Input: dimensioned drawing with shaded views. Units: mm. Origin: part minimum x, y, z. A direction names the side the tool comes from. Give positions to 0.01 mm unless a question says otherwise; leave off trailing zeros. Loops run counter-clockwise (first coordinate to the right, second up) from the corner with the lowest first, then second, coordinate; pieces in that order, holes last.
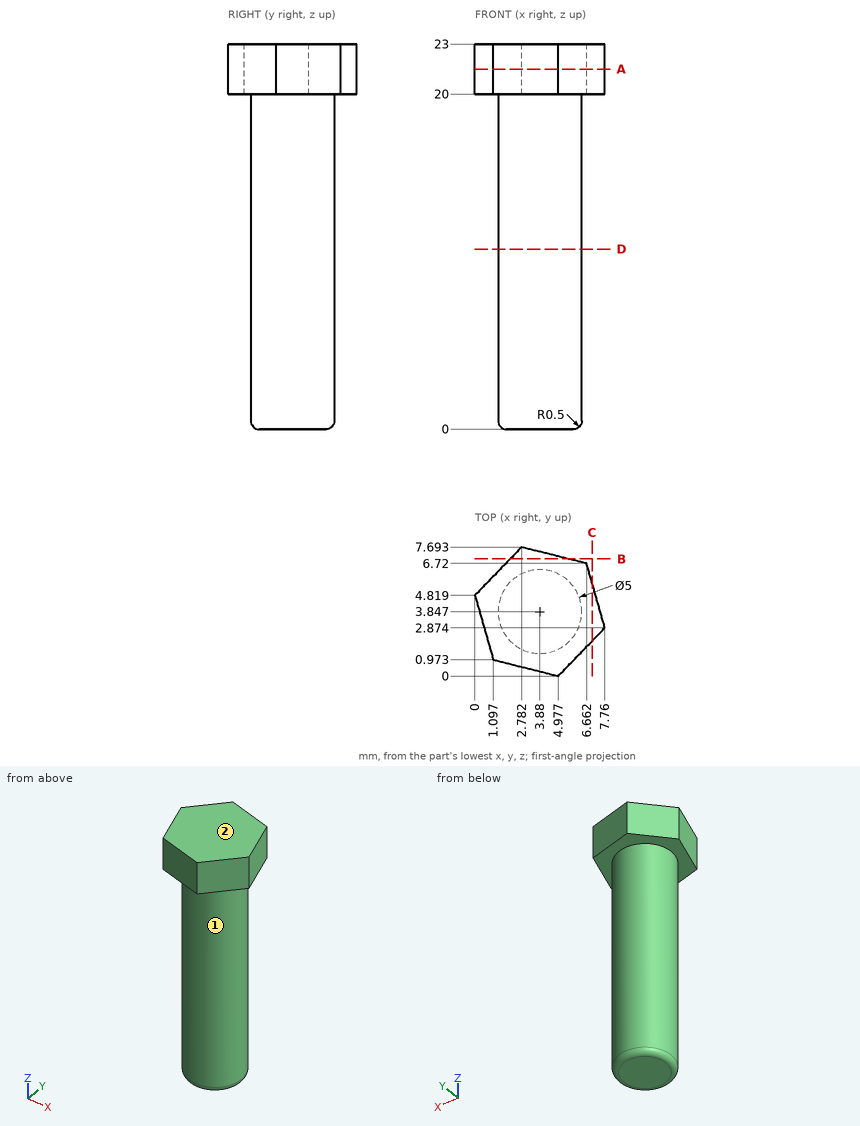
Item 1: Ray query, probe 1 along X at (y, z) = (3.75, 13.5); probe 2 along Z at (x, y) = (7.25, 3); probe 3 along Y at (x, z) = (2, 7.25) (1 decimal). Return the intervals inside material, ascending.
Values follow:
probe 1: x = 1.38 to 6.38
probe 2: z = 20 to 23
probe 3: y = 2.2 to 5.5
Item 2: Section query D-D on z = 10.75. Return loops of the section in (x, y).
Values follow:
outline: circle Ø5 at (3.88, 3.85)
Item 3: Set-up query: the marked faces 1 and 2. Return all of +Z, -Z, +X, -X, +Y, -Y with unobstructed straight access to the full face (end or side cutting, diameter ignored); none if empty.
Values follow:
face 1: -Z
face 2: +Z, +X, -X, +Y, -Y
Item 4: Pin query (flat end, axial travel): pin 1 (1.5 mm diameter, centred on x = 6.5, y = 2.5, fed in from -Z); pin 2 (3 mm diameter, centred on x = 7, z = 14.5, fed in from -Y); pin 3 (4 mm diameter, centred on x = 1, z = 6, fed in from -Y). Return the tip coordinate at first contact, or that it passes through.
Values follow:
pin 1: stops at z = 0.04
pin 2: stops at y = 1.94
pin 3: stops at y = 1.51
Item 5: Section query C-C on x = 7. Return loops of the section in (y, z).
Values follow:
outline: (2.09, 20) - (5.54, 20) - (5.54, 23) - (2.09, 23) - close
Item 6: Section query B-B on y = 7. Return loops of the section in (x, z).
Values follow:
outline: (2.11, 20) - (5.55, 20) - (5.55, 23) - (2.11, 23) - close
Item 7: Section query A-A on z = 21.5. Return loops of the section in (x, y).
Values follow:
outline: (0, 4.82) - (1.1, 0.97) - (4.98, 0) - (7.76, 2.87) - (6.66, 6.72) - (2.78, 7.69) - close
